Could you check a few things on this model? Use its own coordinates, in mm. A direction names the side the tool comes from. Coordinates: 2 decimals unless noted, no trailing zeros. Write each loop counter-clockwise with the first axis right and the second up, starting at its lowest first coordinate (ties: lowest second). Pieces come first, ordered by that corner, then holes. Notation, with made-up numbers: M 82.25,41 L 103.25,41 A26 ccw 103.25,78 Z; hole C -20.75,47.5 d5. An arc over 180 degrees is marked long. Write item = value, one per line.
```python
from build123d import *

# Parameters (mm, degrees)
F0_R     = 3.875
F1_DEPTH = 2.675
F2_R     = 2
F3_R     = 8
F3_R_2   = 3.875
F4_DEPTH = 2.5
F5_R     = 2
F6_R     = 7
F6_R_2   = 3.875
F7_DEPTH = 4


with BuildPart() as f1:
    # F0 (on Front) → F1 (new body, symmetric)
    with BuildSketch(Plane.XZ):
        with BuildLine():
            ThreePointArc((34.3685322209, -3.0420949584), (35.4004522993, 0), (34.3685322209, 3.0420949584))
            ThreePointArc((34.3685322209, 3.0420949584), (0, 20), (-34.3685322209, 3.0420949584))
            ThreePointArc((-34.3685322209, 3.0420949584), (-35.4004522993, 0), (-34.3685322209, -3.0420949584))
            ThreePointArc((-34.3685322209, -3.0420949584), (0, -20), (34.3685322209, -3.0420949584))
        make_face()
        with BuildLine():
            ThreePointArc((-30.4004522993, 0), (-23.1775008297, 7.7461532708), (-14.0563482176, 13.129320875))
            ThreePointArc((-14.0563482176, 13.129320875), (-10.4981429131, 0), (-14.0563482176, -13.129320875))
            ThreePointArc((-14.0563482176, -13.129320875), (-23.1775008297, -7.7461532708), (-30.4004522993, 0))
        make_face(mode=Mode.SUBTRACT)
        Circle(F0_R, mode=Mode.SUBTRACT)
        with BuildLine():
            ThreePointArc((14.0563482176, 13.129320875), (23.1775008297, 7.7461532708), (30.4004522993, 0))
            ThreePointArc((30.4004522993, 0), (23.1775008297, -7.7461532708), (14.0563482176, -13.129320875))
            ThreePointArc((14.0563482176, -13.129320875), (10.4981429131, 0), (14.0563482176, 13.129320875))
        make_face(mode=Mode.SUBTRACT)
    extrude(amount=F1_DEPTH, both=True)

    # F2
    f2_edges = [f1.edges().sort_by_distance(p)[0] for p in [
        (-14.056348, 0, 13.129321),
        (-30.400452, 0, 0),
        (-14.056348, 0, -13.129321),
        (14.056348, 0, 13.129321),
        (30.400452, 0, 0),
        (14.056348, 0, -13.129321),
    ]]
    fillet(f2_edges, radius=F2_R)

    # F3 (on face) → F4 (join)
    with BuildSketch(Plane.XZ.offset(2.675)):
        with BuildLine():
            ThreePointArc((32.7813002522, -1.825256975), (33.4004522993, 0), (32.7813002522, 1.825256975))
            ThreePointArc((32.7813002522, 1.825256975), (0, 18), (-32.7813002522, 1.825256975))
            ThreePointArc((-32.7813002522, 1.825256975), (-33.4004522993, 0), (-32.7813002522, -1.825256975))
            ThreePointArc((-32.7813002522, -1.825256975), (0, -18), (32.7813002522, -1.825256975))
        make_face()
        with BuildLine():
            ThreePointArc((-32.2700519058, 0), (0, 16.5), (32.2700519058, 0))
            ThreePointArc((32.2700519058, 0), (0, -16.5), (-32.2700519058, 0))
        make_face(mode=Mode.SUBTRACT)
        Circle(F3_R)
        Circle(F3_R_2, mode=Mode.SUBTRACT)
    extrude(amount=F4_DEPTH)

    # F5
    f5_edges = [f1.edges().sort_by_distance(p)[0] for p in [
        (-32.270052, -3.925, 0),
        (32.270052, -3.925, 0),
    ]]
    fillet(f5_edges, radius=F5_R)

    # F6 (on face) → F7 (join)
    with BuildSketch(Plane.XZ.offset(5.175)):
        Circle(F6_R)
        Circle(F6_R_2, mode=Mode.SUBTRACT)
    extrude(amount=F7_DEPTH)

    # F8: F1 across plane


with BuildPart() as f1_1:
    add(f1.part)
    add(f1.part.mirror(Plane.XZ))


solid = f1_1.part
```
Item 1: I'm going to push flat-ended pins straight in: P1, Ø3, axis at y = -4, z = -8, coming from the -X side; P2, Ø1.5, axis at x = 6.5, y = 7, coming from the +Z side; P3, Ø3, axis at x = -24.5, y = -0.5, coming from the -Z side. Where does each tip first touch, or does it pass through?
Numbers:
P1 = -30.64
P2 = 3.99
P3 = -13.39
Item 2: For faces 1 (the face through (6.466, 7.147, -2.681)), 2 (the face through (-23.241, -0.037, -7.695)), 3 (the face through (-5, -2.675, -18)), which set-ups out of +Z, -Z, +X, -X, +Y, -Y let a thin tool reach every point of the face, with its end or its side?
Numbers:
face_1 = +Y
face_2 = +Y, -Y
face_3 = -Y
Item 3: If I drill on line 1 along Z through (x, y) = (0, 6.25) (3 decimals); line 2 along X through (y, z) = (-2.5, 2); line 3 along Z through (x, y) = (-3.5, -4.25), over which ranges is the centre line in solid material (lowest first)?
Numbers:
line_1 = -7 to -3.875, 3.875 to 7
line_2 = -34.98 to -28.91, -10.58 to -3.32, 3.32 to 10.58, 28.91 to 34.98
line_3 = -17.85 to -16.35, -7.19 to -1.66, 1.66 to 7.19, 16.35 to 17.85
Item 4: If we mould it in two halves opening along X, with no side actions, what happens to faces 4 (the face through (0.53, 3.907, 17.997)), 5 (the face through (-35.4, 0, 0)), 6 (the face through (10.5, 0, -0.2))? For each: pulls with the +X half, pulls with the -X half, needs draft (parallel to the pull), parting line crosses it, or undercut.
Numbers:
face_4 = parting line crosses it
face_5 = pulls with the -X half
face_6 = undercut
Item 5: Imagine slicing it at B-B (x = -21.5). Write out the boundary of the cut face in (y, z) (3 decimals).
Numbers:
outline = M -5.175,-11.964 L -2.675,-11.964 L -2.675,-14.286 L 2.675,-14.286 L 2.675,-11.964 L 5.175,-11.964 L 5.175,-10.194 L 2.675,-10.194 L 2.675,-9.017 L -2.675,-9.017 L -2.675,-10.194 L -5.175,-10.194 Z; M -5.175,10.194 L -2.675,10.194 L -2.675,9.017 L 2.675,9.017 L 2.675,10.194 L 5.175,10.194 L 5.175,11.964 L 2.675,11.964 L 2.675,14.286 L -2.675,14.286 L -2.675,11.964 L -5.175,11.964 Z
Item 6: Imagine slicing it at D-D (z = 14). Write out the boundary of the cut face in (x, y) (3 decimals), and give its area (3 significant figures).
Numbers:
outline = M -21.993,-2.675 L -17.733,-2.675 L -17.733,-5.175 L -13.885,-5.175 L -13.885,-2.675 L 13.885,-2.675 L 13.885,-5.175 L 17.733,-5.175 L 17.733,-2.675 L 21.993,-2.675 L 21.993,2.675 L 17.733,2.675 L 17.733,5.175 L 13.885,5.175 L 13.885,2.675 L -13.885,2.675 L -13.885,5.175 L -17.733,5.175 L -17.733,2.675 L -21.993,2.675 Z
area = 274 mm²
Item 7: Imagine slicing it at A-A (y = -4.25). State how many separate pieces and enclosed holes the cut face has, and give its area (3 significant figures).
Numbers:
separate_pieces = 2
enclosed_holes = 2
area = 386 mm²
